Job drawing, mm, ordinate dimensions from the low corner. One solid piece. Round coordinates to 2 decimals unless told otherwise and drop trailing zeros. Write each loop counter-clockwise with the first axis right and the second up, starting at its lowest first coordinate (ties: lowest second). Pieces come first, ordered by that corner, then holes.
1) Saw through at A-A on x = 31.75. Write the cut outline in (y, z).
2) Flat gauge pins, fed straight in: pin 1 (6 mm diameter, centred on y = 41, z = 3.5, fed in from -X); pin 2 (10 mm diameter, centred on x = 27.5, z = 11, fed in from +Y); pin 3 (5 mm diameter, centred on y = 52.5, z = 16, fed in from -X). Where does each tip first touch, or does it go through?
3) Saw through at C-C on x = 44. Write the cut outline in (y, z).
4) Saw through at D-D on z = 2.75. Count the separate pieces of the cut face and the enclosed holes in it, and give its area (3 significant figures).
5) Drill centre lines: L1, parallel to Y at x = 31.75, z = 14.5; L2, parallel to Y at x = 31, z = 2; L3, parallel to Y at x = 29.5, z = 4.5. Where is each one in solid material? Low to high.
6) Pull direction Y, two halves, no side cores. Call the marked faces 1, 2 and 3: +Y half, -Y half, draft (parallel to the pull), parting line (faces both ways), or undercut.
7) Saw through at B-B on y = 31.75. Write the cut outline in (x, z), and give its area (3 significant figures).
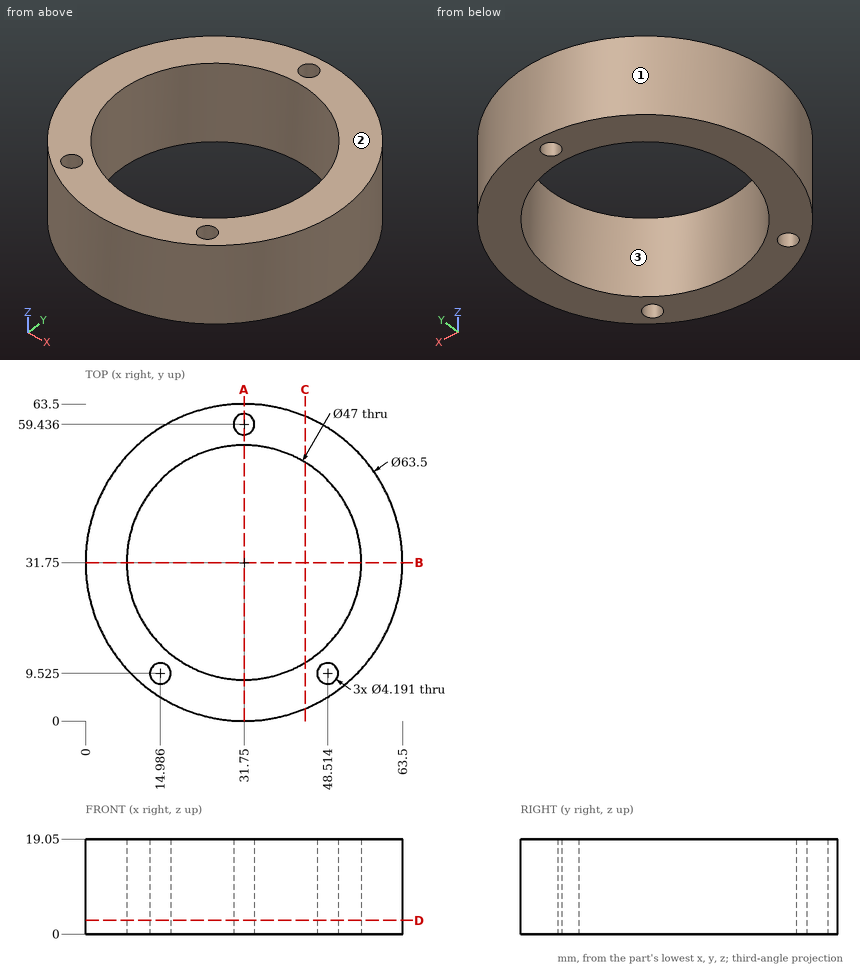
Completed:
1. outline: (0, 0) - (8.25, 0) - (8.25, 19.05) - (0, 19.05) - close; (55.25, 0) - (57.34, 0) - (57.34, 19.05) - (55.25, 19.05) - close; (61.53, 0) - (63.5, 0) - (63.5, 19.05) - (61.53, 19.05) - close
2. pin 1: stops at x = 0.62
2. pin 2: stops at y = 63.5
2. pin 3: stops at x = 5.77
3. outline: (2.46, 0) - (11.7, 0) - (11.7, 19.05) - (2.46, 19.05) - close; (51.8, 0) - (61.04, 0) - (61.04, 19.05) - (51.8, 19.05) - close
4. separate pieces: 1
4. enclosed holes: 4
4. area: 1,390 mm2
5. L1: y = 0 to 8.25, 55.25 to 57.34, 61.53 to 63.5
5. L2: y = 0.01 to 8.26, 55.24 to 57.48, 61.39 to 63.49
5. L3: y = 0.08 to 8.36, 55.14 to 63.42
6. face 1: parting line
6. face 2: draft
6. face 3: undercut
7. outline: (0, 0) - (8.25, 0) - (8.25, 19.05) - (0, 19.05) - close; (55.25, 0) - (63.5, 0) - (63.5, 19.05) - (55.25, 19.05) - close
7. area: 314 mm2
